Verification items for this drawing (mm, ordinates from the low corner). A direction names the side the tool comes from. Coordinates: 2 decimals unless noted, no trailing zeros. Order: outer loops, then holes, each group sorted by start corner. A loop starts at its lowest first (then second) coordinate and runs counter-clockwise, first axis right, second up. Notation, with made-up numbers: (67, 78.5) - (91, 78.5) arc R18 cw to (91, 102.5) - close; hole circle Ø4 at (11, -36.5). An arc over 180 degrees is marked (long way). One line per question, with ' | ' between items. Start each with the question number.
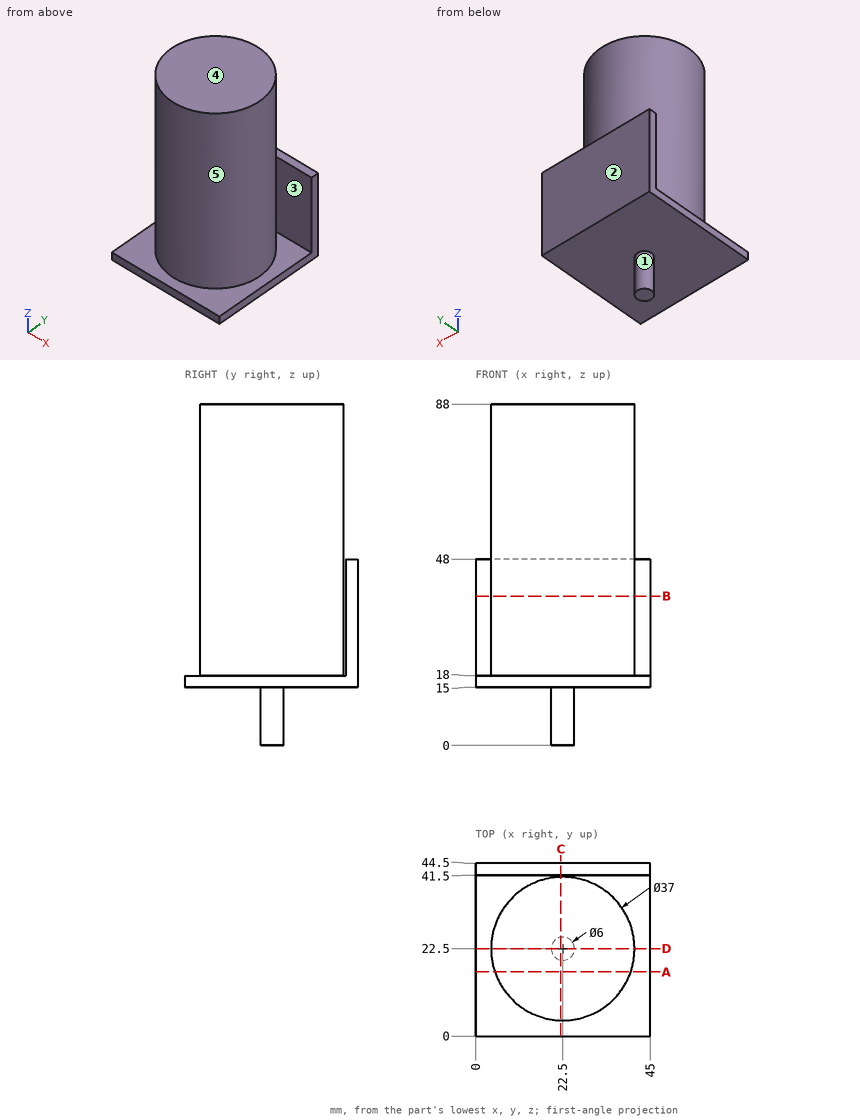
Item 1: Thickness scan on probe 1 along Z at (x, y) = (23, 37.5); probe 2 along Z at (x, y) = (3.5, 38); probe 3 along Y at (x, z) = (8.5, 47). Record the ranges inside material, lowest first. Write a range as from..to.
Item 2: Section check B-B (z = 38.5). Record the cut outline in (x, y), then the cut area to 3 significant figures.
Item 3: Section check D-D (y = 22.5). Record the cut outline in (x, z).
Item 4: Gauge pin test, flat ends, axial feed: pin 1 (3 mm diameter, centred on x = 9, z = 62.5, fed in from -Y); pin 2 (12 mm diameter, centred on x = 15.5, z = 68.5, fed in from +Y); pin 3 (1.5 mm diameter, centred on x = 24.5, z = 44, fed in from -Y). Record the tip position at first contact, or that the pin passes through.
Item 5: Section check A-A (y = 16.5). Record the cut outline in (x, z).
Item 6: Mould release check, pull along Y, two halves, no side actions. Record for the marked faces 1, 2 and 3: +Y half, -Y half, draft (parallel to the pull), parting line (faces both ways), or undercut.
Item 7: Section check C-C (x = 22). Record the cut outline in (y, z).
Item 8: Set-up check for the marked faces 4 and 5: record each of +Z, -Z, +X, -X, +Y, -Y from which the full face is reachable in a straight line by a thin tool's end or side.
Completed:
1) probe 1: z = 15..88 | probe 2: z = 15..18 | probe 3: y = 10.41..34.59, 41.5..44.5
2) outline: (0, 41.5) - (45, 41.5) - (45, 44.5) - (0, 44.5) - close; circle Ø37 at (22.5, 22.5) | area: 1,210 mm^2
3) outline: (0, 15) - (19.5, 15) - (19.5, 0) - (25.5, 0) - (25.5, 15) - (45, 15) - (45, 18) - (41, 18) - (41, 88) - (4, 88) - (4, 18) - (0, 18) - close
4) pin 1: stops at y = 8.42 | pin 2: stops at y = 40.97 | pin 3: stops at y = 4.04
5) outline: (0, 15) - (45, 15) - (45, 18) - (40, 18) - (40, 88) - (5, 88) - (5, 18) - (0, 18) - close
6) face 1: parting line | face 2: +Y half | face 3: undercut
7) outline: (0, 15) - (19.54, 15) - (19.54, 0) - (25.46, 0) - (25.46, 15) - (44.5, 15) - (44.5, 48) - (41.5, 48) - (41.5, 18) - (40.99, 18) - (40.99, 88) - (4.01, 88) - (4.01, 18) - (0, 18) - close
8) face 4: +Z, +X, -X, +Y, -Y | face 5: +Z
